from build123d import *

# Parameters (mm, degrees)
SKETCH1_W           = 50.8
SKETCH1_H           = 50.8
BOSS_EXTRUDE1_DEPTH = 4.572
CUT_EXTRUDE1_DEPTH  = 4.572


with BuildPart() as part:
    # Sketch1 → Boss-Extrude1 (new body)
    with BuildSketch(Plane.XY):
        with Locations((6.5024, -6.366933333)):
            Rectangle(SKETCH1_W, SKETCH1_H)
    extrude(amount=BOSS_EXTRUDE1_DEPTH)

    # Sketch2 → Cut-Extrude1 (cut)
    with BuildSketch(Plane(origin=(0, 0, 0), x_dir=(-1, 0, 0), z_dir=(0, 0, -1))):
        with BuildLine():
            ThreePointArc((7.7851, -6.366933333), (3.600388136, 3.735854803), (-6.5024, 7.920566667))
            Line((-6.5024, 7.920566667), (-6.5024, -6.366933333))
            Line((-6.5024, -6.366933333), (7.7851, -6.366933333))
        make_face()
        with BuildLine():
            Line((-6.5024, -6.366933333), (-6.5024, 7.920566667))
            ThreePointArc((-6.5024, 7.920566667), (-16.605188136, 3.735854803), (-20.7899, -6.366933333))
            Line((-20.7899, -6.366933333), (-6.5024, -6.366933333))
        make_face()
        with BuildLine():
            Line((7.7851, -6.366933333), (-6.5024, -6.366933333))
            Line((-6.5024, -6.366933333), (-6.5024, -20.654433333))
            ThreePointArc((-6.5024, -20.654433333), (3.600388136, -16.46972147), (7.7851, -6.366933333))
        make_face()
        with BuildLine():
            Line((-6.5024, -20.654433333), (-6.5024, -6.366933333))
            Line((-6.5024, -6.366933333), (-20.7899, -6.366933333))
            ThreePointArc((-20.7899, -6.366933333), (-16.605188136, -16.46972147), (-6.5024, -20.654433333))
        make_face()
    extrude(amount=-CUT_EXTRUDE1_DEPTH, mode=Mode.SUBTRACT)


solid = part.part
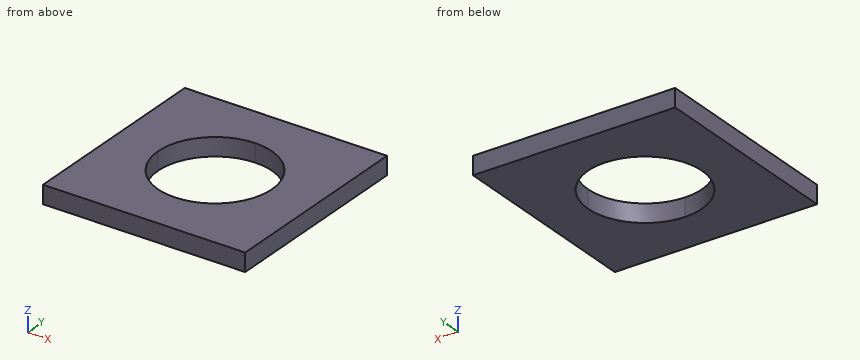
The model under review builds one solid part; all positions refer to its coordinate system, in mm. Coordinates: 2 decimals unless noted, no trailing zeros. Loops run counter-clockwise (first coordinate to the right, second up) from the corner with the lowest first, then second, coordinate; pieces in that order, holes last.
(1) Consider section C-C, the plane x = 5. Give the boundary of the cut face in (y, z).
Determined:
outline: (-31.77, 0) - (-20.58, 0) - (-20.58, 4.57) - (-31.77, 4.57) - close; (7.84, 0) - (19.03, 0) - (19.03, 4.57) - (7.84, 4.57) - close
(2) Wall thickness on L1, parallel to X at y = -5, z = 0.4; L2, parallel to Y at x = 8, z = 2; L3, parallel to Y at x = 16.5, z = 4.1: over which ranges is each line inside the solid? List them lowest first.
Determined:
L1: x = -18.9 to -7.72, 20.72 to 31.9
L2: y = -31.77 to -20.58, 7.84 to 19.03
L3: y = -31.77 to -16.57, 3.84 to 19.03
(3) Consider section B-B, the plane z = 3.5. Give the boundary of the cut face in (x, y) (1 decimal).
Determined:
outline: (-18.9, -31.8) - (31.9, -31.8) - (31.9, 19) - (-18.9, 19) - close; hole circle Ø28.6 at (6.5, -6.4)
(4) Consider section A-A, the plane y = 1. Give the boundary of the cut face in (x, z), plus the area to 3 significant figures.
Determined:
outline: (-18.9, 0) - (-5.74, 0) - (-5.74, 4.57) - (-18.9, 4.57) - close; (18.74, 0) - (31.9, 0) - (31.9, 4.57) - (18.74, 4.57) - close
area: 120 mm2
